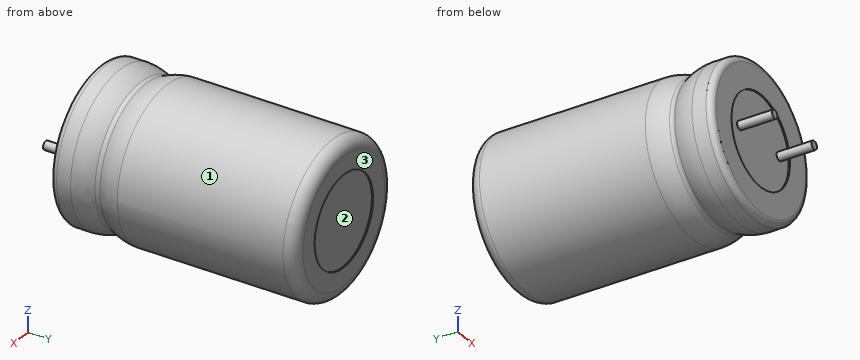
from build123d import *

# Parameters (mm, degrees)
SKETCH2_R                = 0.35
BASE_EXTRUDE_DEPTH       = 3
SKETCH3_R                = 3.75
BOSS_EXTRUDE1_DEPTH      = 0.5
SKETCH4_R                = 0.35
BOSS_EXTRUDE2_DEPTH      = 3
SKETCH5_R                = 6.25
BOSS_EXTRUDE4_DEPTH      = 0.1
BOSS_EXTRUDE4_DEPTH_BACK = 20.2
SKETCH7_R                = 3.75
SKETCH7_R_2              = 0.35
CUT_EXTRUDE3_DEPTH       = 0.1
FILLET1_R                = 0.5
FILLET2_R                = 1
SKETCH8_R                = 3.75
CUT_EXTRUDE4_DEPTH       = 0.1


with BuildPart() as part:
    # Sketch2 → Base-Extrude (new body)
    with BuildSketch(Plane(origin=(0, 0, 0), x_dir=(1, 0, 0), z_dir=(0, 1, 0))):
        Circle(SKETCH2_R)
    extrude(amount=-BASE_EXTRUDE_DEPTH)

    # Sketch3 → Boss-Extrude1 (add)
    with BuildSketch(Plane(origin=(0, 0, 0), x_dir=(-1, 0, 0), z_dir=(0, 1, 0))):
        with Locations((2.54, 0)):
            Circle(SKETCH3_R)
    extrude(amount=BOSS_EXTRUDE1_DEPTH)

    # Sketch4 → Boss-Extrude2 (add)
    with BuildSketch(Plane.XZ):
        with Locations((-5.08, 0)):
            Circle(SKETCH4_R)
    extrude(amount=BOSS_EXTRUDE2_DEPTH)

    # Sketch5 → Boss-Extrude4 (add, two sides)
    with BuildSketch(Plane.XZ.offset(0.1)) as boss_extrude4_sk:
        with Locations((-2.54, 0)):
            Circle(SKETCH5_R)
    extrude(amount=BOSS_EXTRUDE4_DEPTH)
    extrude(boss_extrude4_sk.sketch, amount=-BOSS_EXTRUDE4_DEPTH_BACK)

    # Sketch7 → Cut-Extrude3 (cut)
    with BuildSketch(Plane.XZ.offset(0.2)):
        with Locations((-2.54, 0)):
            Circle(SKETCH7_R)
        with Locations((-5.08, 0)):
            Circle(SKETCH7_R_2, mode=Mode.SUBTRACT)
        Circle(SKETCH7_R_2, mode=Mode.SUBTRACT)
    extrude(amount=-CUT_EXTRUDE3_DEPTH, mode=Mode.SUBTRACT)

    # Fillet1
    fillet1_edges = [part.edges().sort_by_distance(p)[0] for p in [
        (-8.79, -0.2, 0),
    ]]
    fillet(fillet1_edges, radius=FILLET1_R)

    # Fillet2
    fillet2_edges = [part.edges().sort_by_distance(p)[0] for p in [
        (-8.79, 20.1, 0),
    ]]
    fillet(fillet2_edges, radius=FILLET2_R)

    # Sketch8 → Cut-Extrude4 (cut)
    with BuildSketch(Plane(origin=(0, 20.1, 0), x_dir=(-1, 0, 0), z_dir=(0, 1, 0))):
        with Locations((2.54, 0)):
            Circle(SKETCH8_R)
    extrude(amount=-CUT_EXTRUDE4_DEPTH, mode=Mode.SUBTRACT)

    # Sketch10 → Cut-Revolve1 (revolve, cut)
    with BuildSketch(Plane.XY):
        with BuildLine():
            Line((3.71, 5.69), (4.21, 5.69))
            Line((4.21, 5.69), (4.21, 1.11))
            Line((4.21, 1.11), (3.71, 1.11))
            ThreePointArc((3.71, 1.11), (3.618018735, 2.178778092), (3.26, 3.19))
            ThreePointArc((3.26, 3.19), (3.21, 3.4), (3.26, 3.61))
            ThreePointArc((3.26, 3.61), (3.618018735, 4.621221908), (3.71, 5.69))
        make_face()
    revolve(axis=Axis((-2.54, 0.346345216, 0), (0, 1, 0)), mode=Mode.SUBTRACT)


solid = part.part
For this review, take the finished solid that the model builds, in its own axes (mm). Face numbers are marked on the shaded views. Coordinates: 2 decimals unless noted, no trailing zeros. Loops run counter-clockwise (first coordinate to the right, second up) from the corner with the lowest first, then second, coordinate; pieces in that order, holes last. Notation, with made-up numbers: (31, -10.75) - (45, -10.75) arc R12 cw to (45, -1.75) - close; hole circle Ø5 at (-18, -2). An arc over 180 degrees is marked (long way). Use a Markdown table: item, result. Add a question column.
Item 1: We need section A-A (y = 13.25). Give the boundary of the cut face in (x, z), and give its area (3 significant figures).
Item 2: For line 1 (Y direction, x = -4.5, z = -0.75); line 2 (Y direction, x = 1, z = 2); line 3 (Z direction, x = 2.75, y = 11.25), list the stretches that pass through material, from the lowest coordinate up.
Item 3: Mouldability with a two-part tool opening along X and no side actions: class the marked faces 1, 2 and 3 as pulls with the +X half, pulls with the -X half, needs draft (parallel to the pull), parting line crosses it, or undercut.
Item 4: Insertion check: pin 1 Ø2 at (x, y) = (1.5, 0.5) entering from -Z; pin 2 Ø2 at (x, z) = (-3.5, -0.5) entering from -Y; pin 3 Ø1.5 at (y, z) = (12.5, -1) entering from -X (3 decimals). Each pin has a flat end and moves straight along its axis. Give the tip position at first contact, or say it passes through.
Results list:
| question | item | result |
|---|---|---|
| 1 | outline | circle Ø12.5 at (-2.54, 0) |
| 1 | area | 123 mm^2 |
| 2 | line 1 | y = -0.1 to 20 |
| 2 | line 2 | y = -0.2 to 20.1 |
| 2 | line 3 | z = -3.33 to 3.33 |
| 3 | face 1 | parting line crosses it |
| 3 | face 2 | undercut |
| 3 | face 3 | needs draft |
| 4 | pin 1 | stops at z = -5.46 |
| 4 | pin 2 | stops at y = -0.1 |
| 4 | pin 3 | stops at x = -8.785 |
